Source: CAD feature listing. Evaluate the final solid. Frame: model axes, mm. A direction names the side the tool comes from. Round coordinates to 2 decimals unless told otherwise and drop trailing zeros. Loops run counter-clockwise (first coordinate to the right, second up) from the corner with the lowest first, then second, coordinate; pieces in that order, holes last. Notation, with made-up numbers: M 87,-21.75 L 122,-21.75 A21 cw 122,17.25 Z; hole C 29.5,32 d9. An arc over 180 degrees is marked long. Write each question's results on one line, items separated by ' | '. Start each with the question number.
1. Draft query along X for faces 5 (the cylindrical face through (-4.473, 0.986, -25.352)), 6 (the flat face through (-10, 1, 7)), 7 (the flat face through (0, 1, -30.1)). Return one class per face: released by +X, released by -X, zero draft, split by the parting line, or undercut.
2. Section B-B on x = -14.5. Output: boundary loops of the cut face in (y, z), and give its area (3 significant figures).
3. Section C-C on x = -4.95. Output: boundary loops of the cut face in (y, z).
4. Ray query, line 1 (X direction, y = 0.9, z = 20.7); line 2 (Z direction, x = 4.95, y = 1.05); line 3 (X direction, y = 0.5, z = -15). Return the intervals inside material, ascending.
5. Section A-A on z = 20.7. Output: boundary loops of the cut face in (x, y).
6. Set-up query: faces 1 (the flat face through (10, 1, -3)), 2 (the flat face through (-1, 1, -8)), 3 (the flat face through (-15, 1, -8)), 4 (the flat face through (-15, 1, -21)). Return all of +Z, -Z, +X, -X, +Y, -Y with unobstructed straight access to the full face (end or side cutting, diameter ignored); none if empty.
7. Contact query for flat-ended pins moving along their axis: pin 1 Ø0.6 at (y, z) = (0.5, 0.5) entering from -X; pin 2 Ø2.5 at (x, z) = (-14.5, -14.5) entering from +Y; pin 3 Ø0.6 at (x, y) = (-15, 1) entering from +Z. Output: stop coordinate, or through.
8. Section D-D on y = 1.2. Output: boundary loops of the cut face in (x, z).
Autodesk Inventor part; units mm, degrees
ref_plane "YZ Plane" through (0, 0, 0) normal (1, 0, 0) x (0, 1, 0)
ref_plane "XZ Plane" through (0, 0, 0) normal (0, 1, 0) x (-1, 0, 0)
ref_plane "XY Plane" through (0, 0, 0) normal (0, 0, 1) x (1, 0, 0)
sketch "Boceto1" plane through (0, 0, 0) normal (0, 1, 0) x (-1, 0, 0)
  line L0 (0, -30.1) -> (-8.9011, -30.1)
  line L1 (0, -30.1) -> (-10, -30.1)
  line L2 (0, -30.1) -> (10, -30.1)
  line L3 (10, -30.1) -> (10, 23.3)
  line L4 (10, -30.1) -> (63.4, -30.1) construction
  line L5 (10, 23.3) -> (-10, 23.3)
  line L6 (-10, 23.3) -> (-10, -30.1)
  line L7 (-10, 23.3) -> (-10, 20.7)
  line L8 (-10, 20.7) -> (10, 20.7)
  line L9 (0, 20.7) -> (4.95, 20.7)
  line L10 (4.95, 20.7) -> (-4.95, 20.7)
  circle A0 centre (4.95, 20.7) radius 2.2
  circle A1 centre (-4.95, 20.7) radius 2.2
  line L11 (10, 0) -> (5.5615, 0)
  line L12 (-10, -30.1) -> (-10, -27.5)
  circle A2 centre (4.95, -27.5) radius 2.2
  circle A3 centre (-4.95, -27.5) radius 2.2
  circle A4 centre (4.95, 20.7) radius 2.2
  circle A5 centre (-4.95, 20.7) radius 2.2
  line L13 (7.5, -13.5) -> (7.5, -21)
  line L14 (7.5, -21) -> (-5.5, -21)
  line L15 (-5.5, -21) -> (-5.5, -8)
  line L16 (-5.5, -8) -> (7.5, -8)
  line L17 (7.5, -8) -> (7.5, -13.5)
  line L18 (1, -8) -> (1, -21)
  line L19 (-5.5, -14.5) -> (7.5, -14.5)
  line L20 (1, -14.5) -> (14.5, -14.5)
  circle A6 centre (14.5, -14.5) radius 1.5
  line L21 (10, -8) -> (19.2349, -8)
  line L22 (19.2349, -8) -> (19.2349, -21)
  line L23 (19.2349, -21) -> (10, -21)
  point P0 (0, 0)
  dimension "d8" = 53.4
  dimension "d9" = 90
  dimension "d10" = 20
  dimension "d11" = 2.6
  dimension "d12" = 4.95
  dimension "d13" = 9.9
  dimension "d14" = 4.4
  dimension "d15" = 4.4
  dimension "d16" = 2.6
  dimension "d19" = 4.4
  dimension "d20" = 4.4
  dimension "d26" = 13.5
  dimension "d27" = 3
extrude "Extrusión1" add sketch "Boceto1" along normal blind 2 contours L0 L1 L6 L8 A1 A0 L3 L2 | L3 L21 L22 L23 | L6 L5 L3 L8 A0 A1
properties part number "plataforma_nueva"
Taken from the geometry:
1) face 5: undercut | face 6: released by -X | face 7: zero draft
2) outline: M 0,-21 L 2,-21 L 2,-16 L 0,-16 Z; M 0,-13 L 2,-13 L 2,-8 L 0,-8 Z | area: 20.0 mm^2
3) outline: M 0,-30.1 L 2,-30.1 L 2,-29.7 L 0,-29.7 Z; M 0,-25.3 L 2,-25.3 L 2,-21 L 0,-21 Z; M 0,-8 L 2,-8 L 2,18.5 L 0,18.5 Z; M 0,22.9 L 2,22.9 L 2,23.3 L 0,23.3 Z
4) line 1: -10 to -7.15, -2.75 to 2.75, 7.15 to 10 | line 2: -30.1 to -29.7, -25.3 to -21, -8 to 18.5, 22.9 to 23.3 | line 3: -19.23 to -15.91, -13.09 to -7.5, 5.5 to 10
5) outline: M -10,0 L -7.15,0 L -7.15,2 L -10,2 Z; M -2.75,0 L 2.75,0 L 2.75,2 L -2.75,2 Z; M 7.15,0 L 10,0 L 10,2 L 7.15,2 Z
6) face 1: +Z, -Z, +X, +Y, -Y | face 2: +Y, -Y | face 3: +Z, -X, +Y, -Y | face 4: -Z, -X, +Y, -Y
7) pin 1: x = -10 | pin 2: through | pin 3: z = -8
8) outline: M -19.23,-21 L -10,-21 L -10,-30.1 L 10,-30.1 L 10,23.3 L -10,23.3 L -10,-8 L -19.23,-8 Z; hole C -14.5,-14.5 d3; hole M -7.5,-21 L 5.5,-21 L 5.5,-8 L -7.5,-8 Z; hole C -4.95,-27.5 d4.4; hole C -4.95,20.7 d4.4; hole C 4.95,-27.5 d4.4; hole C 4.95,20.7 d4.4
